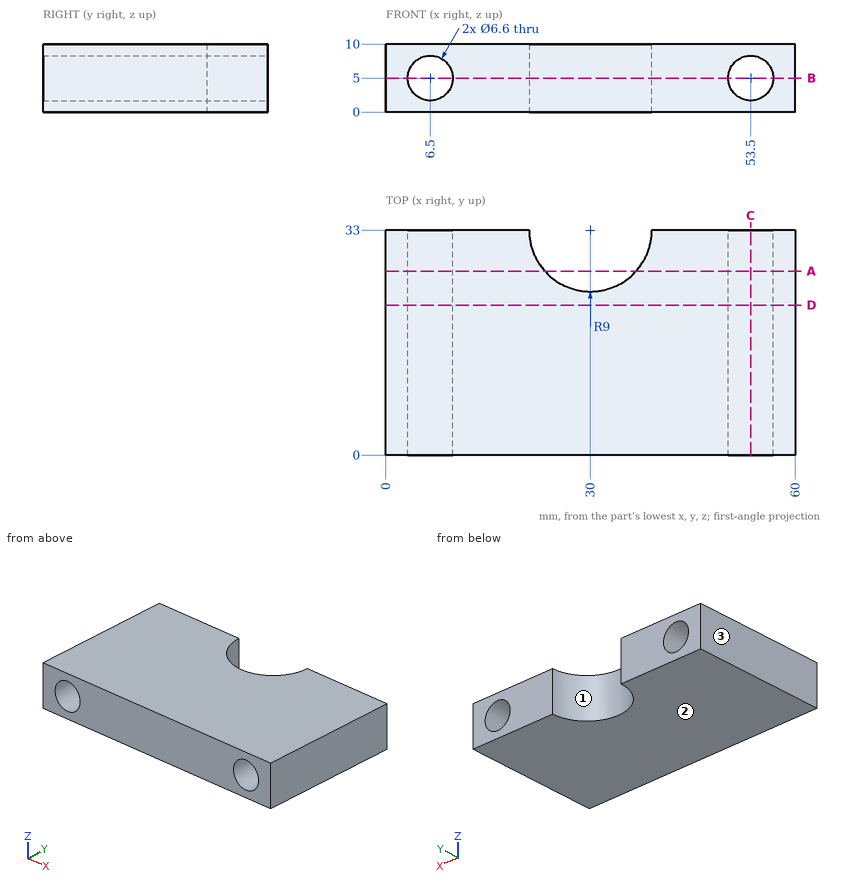
Geometry: see drawing. Coordinates: mm, zero at the bounding-box minimum. Round coordinates to 2 decimals unless told otherwise and drop trailing zeros. Write each loop counter-clockwise with the first axis right and the second up, starting at its lowest first coordinate (ties: lowest second). Pieces come first, ordered by that corner, then holes.
Item 1: Section query B-B (z = 5). Return loops of the section in (x, y), plus the area to 3 significant figures.
Item 2: Material intervals for L1, parallel to X at y = 13, z = 5; L2, parallel to X at y = 32.5, z = 7.75; L3, parallel to X at y = 18.5, z = 6.5, sorted ascending.
Item 3: Section query D-D (y = 22). Return loops of the section in (x, z).
Item 4: Section query C-C (x = 53.5). Return loops of the section in (y, z).
Item 5: Pin query (flat end, axial travel): P1, Ø5.5, axis at x = 6.5, z = 5, coming from the +Y side. Return the tip coordinate at first contact, or that it passes through.
Item 6: Section query A-A (y = 27). Return loops of the section in (x, z), plus the area to 3 significant figures.
Item 7: Mould query, pull axis X, two halves, no side actions, for the marked faces 1, 2 and 3. Classes: +X half, -X half, draft (parallel to the pull), parting line (faces both ways), or undercut.
Completed:
1. outline: (0, 0) - (3.2, 0) - (3.2, 33) - (0, 33) - close; (9.8, 0) - (50.2, 0) - (50.2, 33) - (39, 33) arc R9 cw to (21, 33) - (9.8, 33) - close; (56.8, 0) - (60, 0) - (60, 33) - (56.8, 33) - close
1. area: 1,420 mm2
2. L1: x = 0 to 3.2, 9.8 to 50.2, 56.8 to 60
2. L2: x = 0 to 4.68, 8.32 to 21.01, 38.99 to 51.68, 55.32 to 60
2. L3: x = 0 to 3.56, 9.44 to 50.56, 56.44 to 60
3. outline: (0, 0) - (60, 0) - (60, 10) - (0, 10) - close; hole circle Ø6.6 at (6.5, 5); hole circle Ø6.6 at (53.5, 5)
4. outline: (0, 0) - (33, 0) - (33, 1.7) - (0, 1.7) - close; (0, 8.3) - (33, 8.3) - (33, 10) - (0, 10) - close
5. P1: passes through
6. outline: (0, 0) - (23.29, 0) - (23.29, 10) - (0, 10) - close; (36.71, 0) - (60, 0) - (60, 10) - (36.71, 10) - close; hole circle Ø6.6 at (6.5, 5); hole circle Ø6.6 at (53.5, 5)
6. area: 397 mm2
7. face 1: undercut
7. face 2: draft
7. face 3: -X half
